from build123d import *

# Parameters (mm, degrees)
SKETCH2_W               = 90
SKETCH2_H               = 120
BOSS_EXTRUDE1_DEPTH     = 31.5
SKETCH4_W               = 87
SKETCH4_H               = 117
CUT_EXTRUDE1_DEPTH      = 30
FILLET4_R               = 4
SKETCH18_W              = 57
SKETCH18_H              = 53.6
KHAY_PIN_DEPTH          = 12.5
SKETCH21_W              = 53
SKETCH21_H              = 49.6
BOSS_EXTRUDE11_DEPTH    = 15
SKETCH22_W              = 53
SKETCH22_H              = 49.6
CUT_EXTRUDE4_DEPTH      = 13.5
SKETCH30_W              = 7
SKETCH30_H              = 14
CUT_EXTRUDE8_DEPTH      = 5
SKETCH34_R              = 4.242640687
BOSS_EXTRUDE12_DEPTH    = 7
SKETCH37_W              = 7.9
SKETCH37_H              = 15.9
CUT_EXTRUDE10_DEPTH     = 5
MIRROR2_COPY_1_SKETCH_R = 4.242640687
MIRROR2_COPY_1_DEPTH    = 7
SKETCH38_R              = 10
CUT_EXTRUDE11_DEPTH     = 10


with BuildPart() as part:
    # Sketch2 → Boss-Extrude1 (new body)
    with BuildSketch(Plane.XY):
        Rectangle(SKETCH2_W, SKETCH2_H)
    extrude(amount=BOSS_EXTRUDE1_DEPTH)

    # Sketch4 → Cut-Extrude1 (cut)
    with BuildSketch(Plane.XY.offset(31.5)):
        Rectangle(SKETCH4_W, SKETCH4_H)
    extrude(amount=-CUT_EXTRUDE1_DEPTH, mode=Mode.SUBTRACT)

    # Fillet4
    fillet4_edges = [part.edges().sort_by_distance(p)[0] for p in [
        (45, -60, 15.75),
        (-45, -60, 15.75),
        (-45, 60, 15.75),
        (45, 60, 15.75),
    ]]
    fillet(fillet4_edges, radius=FILLET4_R)

    # Sketch18 → khay_pin (add)
    with BuildSketch(Plane.XY.offset(1.5)):
        with Locations((0, -21.775547075)):
            Rectangle(SKETCH18_W, SKETCH18_H)
    extrude(amount=KHAY_PIN_DEPTH)

    # Sketch21 → Boss-Extrude11 (add)
    with BuildSketch(Plane.XY.offset(14)):
        with Locations((0, -21.775547075)):
            Rectangle(SKETCH21_W, SKETCH21_H)
    extrude(amount=-BOSS_EXTRUDE11_DEPTH)

    # Sketch22 → Cut-Extrude4 (cut)
    with BuildSketch(Plane(origin=(0, 0, -1), x_dir=(-1, 0, 0), z_dir=(0, 0, -1))):
        with Locations((0, -21.775547075)):
            Rectangle(SKETCH22_W, SKETCH22_H)
    extrude(amount=-CUT_EXTRUDE4_DEPTH, mode=Mode.SUBTRACT)

    # Sketch30 → Cut-Extrude8 (cut)
    with BuildSketch(Plane.ZY.offset(-26.5)):
        with Locations((9, -8.975547075)):
            Rectangle(SKETCH30_W, SKETCH30_H)
    extrude(amount=-CUT_EXTRUDE8_DEPTH, mode=Mode.SUBTRACT)

    # Sketch34 → Boss-Extrude12 (add)
    with BuildSketch(Plane.XY.offset(31.5)):
        with Locations((-40.5, 55.5)):
            Circle(SKETCH34_R)
    boss_extrude12 = extrude(amount=-BOSS_EXTRUDE12_DEPTH)

    # Sketch37 → Cut-Extrude10 (cut)
    with BuildSketch(Plane(origin=(45, 0, 0), x_dir=(0, 0, -1), z_dir=(1, 0, 0))):
        with Locations((-18.5, 28)):
            Rectangle(SKETCH37_W, SKETCH37_H)
    extrude(amount=-CUT_EXTRUDE10_DEPTH, mode=Mode.SUBTRACT)

    # Mirror1: Boss-Extrude12 across plane
    add(boss_extrude12.mirror(Plane(origin=(0, 0, 0), x_dir=(0, 0, 1), z_dir=(1, 0, 0))))

    # Mirror2: Boss-Extrude12 across plane
    add(boss_extrude12.mirror(Plane.ZX))

    # Mirror2 copy 1 sketch → Mirror2 copy 1 (add)
    with BuildSketch(Plane(origin=(0, 0, 31.5), x_dir=(-1, 0, 0), z_dir=(0, 0, 1))):
        with Locations((-40.5, 55.5)):
            Circle(MIRROR2_COPY_1_SKETCH_R)
    extrude(amount=-MIRROR2_COPY_1_DEPTH)

    # Sketch38 → Cut-Extrude11 (cut)
    with BuildSketch(Plane.XY.offset(14)):
        with Locations((0, -21.775547075)):
            Circle(SKETCH38_R)
    extrude(amount=-CUT_EXTRUDE11_DEPTH, mode=Mode.SUBTRACT)


solid = part.part
Model file for the job. Use its own axes, mm. A direction names the side the tool comes from. Round coordinates to 2 decimals unless told otherwise and drop trailing zeros. Loops run counter-clockwise (first coordinate to the right, second up) from the corner with the lowest first, then second, coordinate; pieces in that order, holes last. Notation, with made-up numbers: M 26.5,-28.5 L 80.5,-28.5 A29 ccw 80.5,6.5 Z; hole C 19.5,-3 d7. An arc over 180 degrees is marked long. One line per question, with ' | ' between items.
1) Band-saw the part on A-A (x = 0). Give the cut face in (y, z).
Solved:
outline: M -60,0 L -46.58,0 L -46.58,12.5 L -31.78,12.5 L -31.78,14 L -48.58,14 L -48.58,1.5 L -58.5,1.5 L -58.5,31.5 L -60,31.5 Z; M -11.78,12.5 L 3.02,12.5 L 3.02,0 L 60,0 L 60,31.5 L 58.5,31.5 L 58.5,1.5 L 5.02,1.5 L 5.02,14 L -11.78,14 Z
2) Band-saw the part on C-C (z = 21). Give the cut face in (x, y).
Solved:
outline: M -45,-56 A4 ccw -41,-60 L 41,-60 A4 ccw 45,-56 L 45,20.05 L 43.5,20.05 L 43.5,-58.5 L -43.5,-58.5 L -43.5,58.5 L 43.5,58.5 L 43.5,35.95 L 45,35.95 L 45,56 A4 ccw 41,60 L -41,60 A4 ccw -45,56 Z
3) Band-saw the part on D-D (x = -20). Give the cut face in (y, z).
Solved:
outline: M -60,0 L -46.58,0 L -46.58,12.5 L 3.02,12.5 L 3.02,0 L 60,0 L 60,31.5 L 58.5,31.5 L 58.5,1.5 L 5.02,1.5 L 5.02,14 L -48.58,14 L -48.58,1.5 L -58.5,1.5 L -58.5,31.5 L -60,31.5 Z
4) Drill centre lines: line 1 along Y through (x, z) = (23.5, 3); line 2 along X through (y, z) = (-9.5, 6.5); line 3 along Y through (x, z) = (0, 12.95). Where is each one in solid material? Low to high.
Solved:
line 1: y = -60 to -58.5, -48.58 to -46.58, 3.02 to 5.02, 58.5 to 60 | line 2: x = -45 to -43.5, -28.5 to -26.5, 43.5 to 45 | line 3: y = -60 to -58.5, -48.58 to -31.78, -11.78 to 5.02, 58.5 to 60
5) Band-saw the part on B-B (y = 24.5). Give the cut face in (x, z), then the cut area to 3 significant figures.
Solved:
outline: M -45,0 L 45,0 L 45,14.55 L 43.5,14.55 L 43.5,1.5 L -43.5,1.5 L -43.5,31.5 L -45,31.5 Z; M 43.5,22.45 L 45,22.45 L 45,31.5 L 43.5,31.5 Z | area: 213 mm²
6) Flat gauge pin, fed straight in: pin 1 (12 mm diameter, centred on x = 35.5, y = -24, fed in from +Z). Where does the tip first touch, or does it go through?
Solved:
pin 1: stops at z = 1.5
7) 3-axis set-ups, long thin cutter, end or side, ignore diameter. For faces 4 (the flat face through (-1, 14, 0)), 5 (the flat face through (40, 55, 24.5)), 6 (the flat face through (26.5, -22, 6)), 7 (the cylindrical face through (-43.859, 58.797, 15.97)), 8 (the flat face through (-28.5, -22, 8)): which of +Z, -Z, +X, -X, +Y, -Y reach the whole face in a straight line?
Solved:
face 4: -Z, +X, -X, +Y, -Y | face 5: none | face 6: -Z | face 7: +Z, -Z, -X, +Y | face 8: +Z
8) Mould opens along X. For faces 1 (the flat face through (40, -55, 24.5)), 2 (the flat face through (-1, -60, 16)), 3 (the cylindrical face through (43.797, 58.859, 15.97)) say: +X half, -X half, draft (parallel to the pull), parting line (faces both ways), or undercut.
Solved:
face 1: undercut | face 2: draft | face 3: +X half
